Verification items for the finished model (mm, model axes). Face numbers are marked on the shaded views. Round coordinates to 2 decimals unless told otherwise and drop trailing zeros. Order: outer loops, then holes, each group sorted by start corner. A loop starts at its lowest first (then second) coordinate and runs counter-clockwise, first axis right, second up. Notation, with made-up numbers: (67, -34.75) -> (103, -34.75) arc R35 cw to (103, -0.75) -> close; hole circle Ø2 at (-35, -3). An arc over 180 degrees is marked (long way). Write item = value, one per line. Start each with the question number.
from build123d import *

# Parameters (mm, degrees)
SKETCH2_W                                = 160
SKETCH2_H                                = 114
BOSS_EXTRUDE1_DEPTH                      = 5
FILLET1_R                                = 3
BOSS_EXTRUDE2_DEPTH                      = 2
MIRROR1_AT_THE_SECOND_PLANE_COPY_1_DEPTH = 2


with BuildPart() as part:
    # Sketch2 → Boss-Extrude1 (new body)
    with BuildSketch(Plane.XY):
        Rectangle(SKETCH2_W, SKETCH2_H)
    extrude(amount=BOSS_EXTRUDE1_DEPTH)

    # Fillet1
    fillet1_edges = [part.edges().sort_by_distance(p)[0] for p in [
        (80, 0, 5),
        (0, -57, 5),
        (-80, 0, 5),
        (-80, -57, 2.5),
        (80, -57, 2.5),
        (80, 57, 2.5),
        (-80, 57, 2.5),
        (0, 57, 5),
    ]]
    fillet(fillet1_edges, radius=FILLET1_R)

    # Sketch5 → Boss-Extrude2 (add)
    with BuildSketch(Plane(origin=(0, 0, 0), x_dir=(-1, 0, 0), z_dir=(0, 0, -1))):
        with BuildLine():
            Line((-60.75, 57), (-80, 37))
            Line((-80, 37), (-80, 54))
            ThreePointArc((-80, 54), (-79.121320344, 56.121320344), (-77, 57))
            Line((-77, 57), (-60.75, 57))
        make_face()
    boss_extrude2 = extrude(amount=BOSS_EXTRUDE2_DEPTH)

    # Sketch7 → Ø3.0mm Dowel Hole1 (revolve, cut)
    with BuildSketch(Plane(origin=(72.49, 50.17, -2), x_dir=(0, 1, 0), z_dir=(1, 0, 0))):
        Polygon((0, 0), (0, 7.151506083), (1.75, 6.1), (1.75, 0), align=None)
    f_3_0mm_dowel_hole1 = revolve(axis=Axis((72.49, 50.17, -8.35), (0, 0, 1)), mode=Mode.SUBTRACT)

    # Mirror1: Boss-Extrude2, Ø3.0mm Dowel Hole1 across plane
    add(boss_extrude2.mirror(Plane.ZX))
    add(f_3_0mm_dowel_hole1.mirror(Plane.ZX), mode=Mode.SUBTRACT)

    # Mirror1 at the second plane: Boss-Extrude2, Ø3.0mm Dowel Hole1 across plane
    add(boss_extrude2.mirror(Plane(origin=(0, 0, 0), x_dir=(0, 0, 1), z_dir=(1, 0, 0))))
    add(f_3_0mm_dowel_hole1.mirror(Plane(origin=(0, 0, 0), x_dir=(0, 0, 1), z_dir=(1, 0, 0))), mode=Mode.SUBTRACT)

    # Mirror1 at the second plane copy 1 sketc → Mirror1 at the second plane copy 1 (add)
    with BuildSketch(Plane(origin=(0, 0, 0), x_dir=(1, 0, 0), z_dir=(0, 0, -1))):
        with BuildLine():
            Line((-60.75, 57), (-80, 37))
            Line((-80, 37), (-80, 54))
            ThreePointArc((-80, 54), (-79.121320344, 56.121320344), (-77, 57))
            Line((-77, 57), (-60.75, 57))
        make_face()
    extrude(amount=MIRROR1_AT_THE_SECOND_PLANE_COPY_1_DEPTH)

    # Mirror1 at the second plane copy 2 sketc → Mirror1 at the second plane copy 2 (revolve, cut)
    with BuildSketch(Plane(origin=(-72.49, -50.17, -2), x_dir=(0, -1, 0), z_dir=(-1, 0, 0))):
        Polygon((0, 0), (0, 7.151506083), (1.75, 6.1), (1.75, 0), align=None)
    revolve(axis=Axis((-72.49, -50.17, -8.35), (0, 0, 1)), mode=Mode.SUBTRACT)


solid = part.part
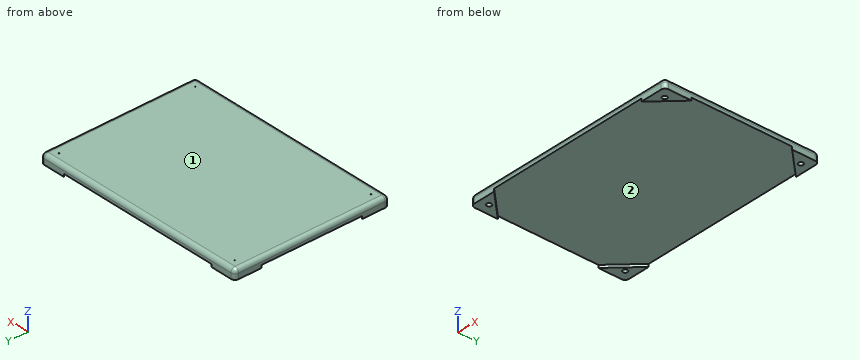
(1) Scan lines: line 1 along X through (y, z) = (-50.17, 0.25); line 2 along Y through (x, z) = (-72.49, 0.25); line 3 along X through (y, z) = (-50.17, 3). Record each from-to range of solid material in increasing order. Write a range as from..to.
(2) Cross-section at A-A (y = -6.5). Enter the section's corners in (x, z), and give its area (3 significant figures).
(3) Cross-section at C-C (y = -46.5). Enter the section's corners in (x, z), and give its area (3 significant figures).
(4) Draft check along X on the marked faces 1 and 2. Enter one of: +X half, -X half, draft (parallel to the pull), parting line (faces both ways), or undercut.
(5) Depth check by flat-ended pin: pin 1 (8 mm diameter, centred on x = -46, y = -31, fed in from -Z); pin 2 (2 mm diameter, centred on y = 37, z = 4, fed in from -X). Enter the tip coordinate at first touch or a pass-through.
(6) Cross-section at B-B (x = 2). Enter the section's corners in (y, z).
Outcome:
q1.line_1 = -80..-74.24, -70.74..70.74, 74.24..80
q1.line_2 = -57..-51.92, -48.42..48.42, 51.92..57
q1.line_3 = -79.83..-74.24, -70.74..70.74, 74.24..79.83
q2.outline = (-80, 0) -> (80, 0) -> (80, 2) arc R3 ccw to (77, 5) -> (-77, 5) arc R3 ccw to (-80, 2) -> close
q2.area = 796 mm^2
q3.outline = (-80, -2) -> (-70.86, -2) -> (-70.86, 0) -> (70.86, 0) -> (70.86, -2) -> (80, -2) -> (80, 2) arc R3 ccw to (77, 5) -> (-77, 5) arc R3 ccw to (-80, 2) -> close
q3.area = 833 mm^2
q4.face_1 = draft
q4.face_2 = undercut
q5.pin_1 = 0
q5.pin_2 = -79.83
q6.outline = (-57, 0) -> (57, 0) -> (57, 2) arc R3 ccw to (54, 5) -> (-54, 5) arc R3 ccw to (-57, 2) -> close
